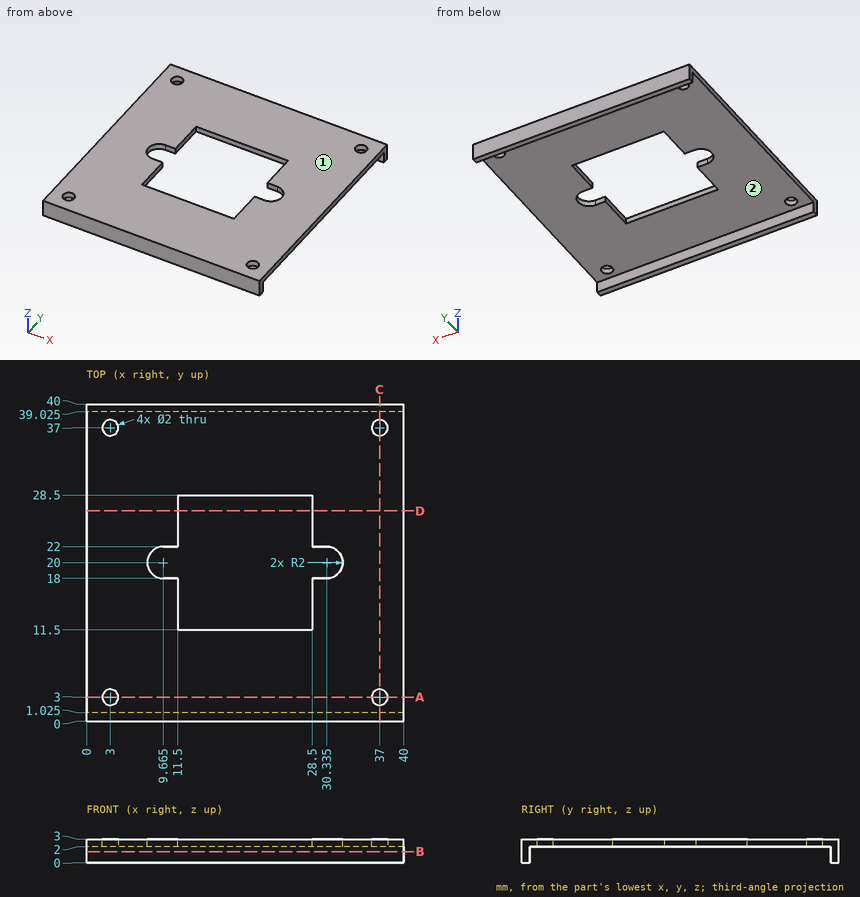
Geometry: see drawing. Coordinates: mm, zero at the bounding-box minimum. Round coordinates to 2 decimals unless told otherwise and drop trailing zeros. Loops run counter-clockwise (first coordinate to the right, second up) from the corner with the lowest first, then second, coordinate; pieces in that order, holes last. Notation, with made-up numbers: M 36.25,82 L 42.25,82 A31 ccw 42.25,107 Z; hole C 14,78 d9. An arc over 180 degrees is marked long. Use a Markdown table: item, result. Add a question column.
1. Cut plane B-B, the plane z = 1.4. Output: boundary loops of the cut face in (x, y) (3 decimals), and give its area (3 significant figures).
2. Contact query for flat-ended pins moving along their axis: pin 1 (1.6 mm diameter, centred on x = 3, y = 37, fed in from +Z); pin 2 (8 mm diameter, centred on x = 17.5, y = 5.5, fed in from -Z). Output: stop coordinate, or through.
3. Ray query, line 1 along Y through (x, z) = (37, 2.7); line 2 along Y through (x, z) = (28, 0.5) (3 decimals); line 3 along Z through (x, y) = (14.5, 5). Return the intervals inside material, ascending. Write a range as [from, to].
4. Cut plane A-A, the plane y = 3. Output: boundary loops of the cut face in (x, z).
5. Cut plane C-C, the plane x = 37. Output: boundary loops of the cut face in (y, z) (3 decimals).
6. Cut plane D-D, the plane y = 26.5. Output: boundary loops of the cut face in (x, z).
7. Pull-direction query (Y, two-part tool) for the marked faces 1 and 2; classes: +Y half, -Y half, draft (parallel to the pull), parting line (faces both ways), or undercut.
Solution:
| question | item | result |
|---|---|---|
| 1 | outline | M 0,0 L 40,0 L 40,1.025 L 0,1.025 Z; M 0,39.025 L 40,39.025 L 40,40 L 0,40 Z |
| 1 | area | 80.0 mm2 |
| 2 | pin 1 | passes through |
| 2 | pin 2 | stops at z = 2 |
| 3 | line 1 | y = [0, 2], [4, 36], [38, 40] |
| 3 | line 2 | y = [0, 1.025], [39.025, 40] |
| 3 | line 3 | z = [2, 3] |
| 4 | outline | M 0,2 L 2,2 L 2,3 L 0,3 Z; M 4,2 L 36,2 L 36,3 L 4,3 Z; M 38,2 L 40,2 L 40,3 L 38,3 Z |
| 5 | outline | M 0,0 L 1.025,0 L 1.025,2 L 2,2 L 2,3 L 0,3 Z; M 4,2 L 36,2 L 36,3 L 4,3 Z; M 38,2 L 39.025,2 L 39.025,0 L 40,0 L 40,3 L 38,3 Z |
| 6 | outline | M 0,2 L 11.5,2 L 11.5,3 L 0,3 Z; M 28.5,2 L 40,2 L 40,3 L 28.5,3 Z |
| 7 | face 1 | draft |
| 7 | face 2 | undercut |
